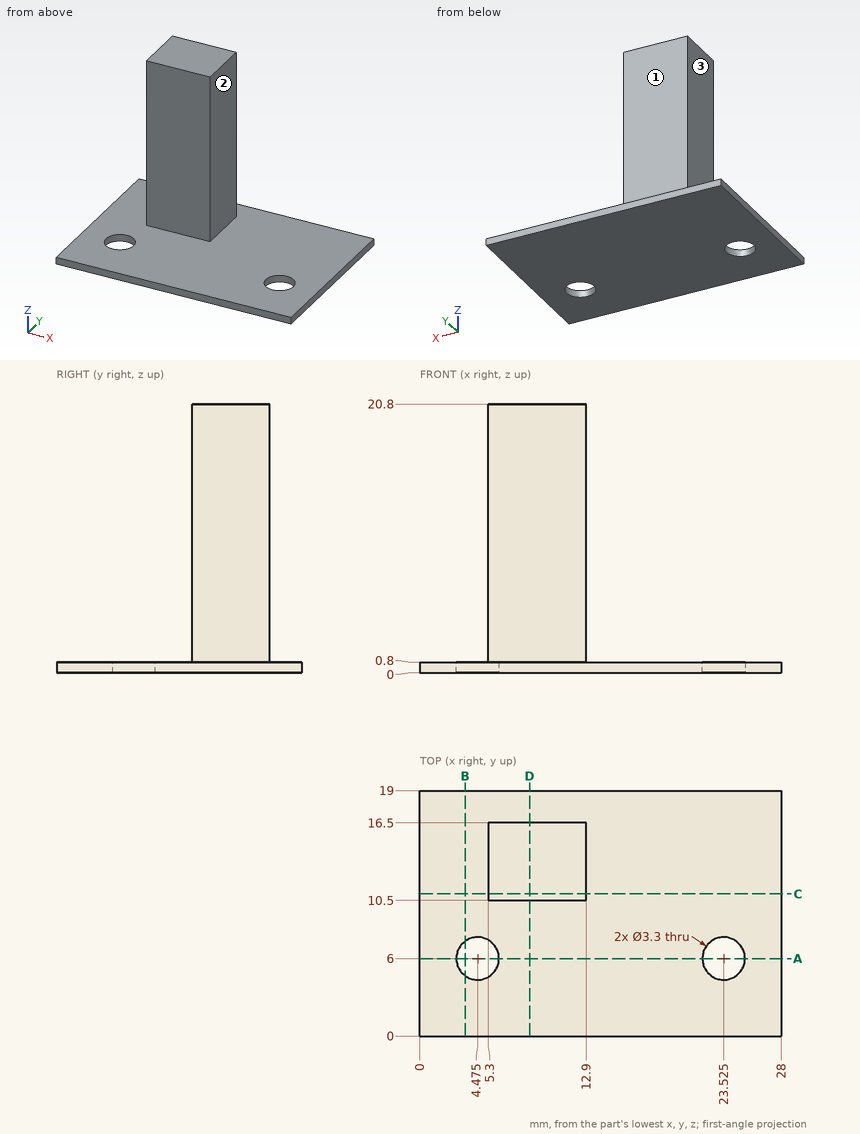
Could you check a few things on this drawing? It's one solid part, dimensions in mm from its lowest x, y, z. A direction names the side the tool comes from. Give positions to 0.01 mm unless a question says otherwise; leave off trailing zeros. Write each loop counter-clockwise with the first axis right and the second up, starting at its lowest first coordinate (ties: lowest second). Pieces come first, ordered by that corner, then holes. Notation, with made-up numbers: (-7, 20.5) - (15, 20.5) arc R15 cw to (15, 45.5) - close; hole circle Ø1 at (-20, 69.25). An arc over 180 degrees is marked (long way). Use CSV: the item, a comma, the result in double quotes. Start each with the question number.
Item 1: I want a section at D-D, the plane x = 8.5. Please give me the cut outline in (y, z), then the cut area to 3 significant figures.
Item 2: I want a section at B-B, the plane x = 3.5. Please give me the cut outline in (y, z), then the cut area to 3 significant figures.
Item 3: I want a section at C-C, the plane y = 11. Please give me the cut outline in (x, z).
Item 4: I'm going to push flat-ended pins straight in: pin 1 (5.5 mm diameter, centred on x = 4.475, y = 6, fed in from -Z); pin 2 (6 mm diameter, centred on y = 12, z = 14, fed in from -X); pin 3 (1 mm diameter, centred on x = 7, z = 15, fed in from -Y); pin 4 (2 mm diameter, centred on x = 6.5, y = 5.5, fed in from +Z). Where does each tip first touch, or does it pass through?
Item 5: If I drill on line 1 along X through (y, z) = (11.5, 17.5); line 2 along Z through (x, y) = (19.75, 4); line 3 along Y through (x, z) = (7.75, 2.5), over which ranges is the centre line in solid material (lowest first)?
Item 6: I want a section at A-A, the plane y = 6. Please give me the cut outline in (x, z) (3 decimals), then the cut area to 3 significant figures.
Item 7: For the marked faces 1, 2 and 3, which set-ups out of +Z, -Z, +X, -X, +Y, -Y let a thin tool reach every point of the face, with its end or its side?
Findings:
1,outline,"(0, 0) - (19, 0) - (19, 0.8) - (16.5, 0.8) - (16.5, 20.8) - (10.5, 20.8) - (10.5, 0.8) - (0, 0.8) - close"
1,area,"135 mm2"
2,outline,"(0, 0) - (4.67, 0) - (4.67, 0.8) - (0, 0.8) - close; (7.33, 0) - (19, 0) - (19, 0.8) - (7.33, 0.8) - close"
2,area,"13.1 mm2"
3,outline,"(0, 0) - (28, 0) - (28, 0.8) - (12.9, 0.8) - (12.9, 20.8) - (5.3, 20.8) - (5.3, 0.8) - (0, 0.8) - close"
4,pin 1,"stops at z = 0"
4,pin 2,"stops at x = 5.3"
4,pin 3,"stops at y = 10.5"
4,pin 4,"stops at z = 0.8"
5,line 1,"x = 5.3 to 12.9"
5,line 2,"z = 0 to 0.8"
5,line 3,"y = 10.5 to 16.5"
6,outline,"(0, 0) - (2.825, 0) - (2.825, 0.8) - (0, 0.8) - close; (6.125, 0) - (21.875, 0) - (21.875, 0.8) - (6.125, 0.8) - close; (25.175, 0) - (28, 0) - (28, 0.8) - (25.175, 0.8) - close"
6,area,"17.1 mm2"
7,face 1,"+Z, +X, -X, +Y"
7,face 2,"+Z, +X, +Y, -Y"
7,face 3,"+Z, -X, +Y, -Y"
